from build123d import *

# Parameters (mm, degrees)
SKETCH_1_R      = 3
SKETCH_1_R_2    = 2
EXTRUDE_1_DEPTH = 3
FILLET_1_R      = 10
SKETCH_2_R      = 4
SKETCH_2_R_2    = 2
EXTRUDE_2_DEPTH = 10


with BuildPart() as part:
    # Эскиз1 → Бобышка-Вытянуть1 (new body)
    with BuildSketch(Plane.XY):
        with BuildLine():
            Line((-17.816178594, -6), (0, -6))
            ThreePointArc((0, -6), (6, 0), (0, 6))
            Line((0, 6), (-20, 6))
            ThreePointArc((-20, 6), (-22.05212086, 5.638155725), (-23.856725658, 4.596266659))
            Line((-23.856725658, 4.596266659), (-36.879481191, -6.331122706))
            ThreePointArc((-36.879481191, -6.331122706), (-37.619022192, -14.784115023), (-29.166029875, -15.523656023))
            Line((-29.166029875, -15.523656023), (-17.816178594, -6))
        make_face()
        with Locations((-20, 0)):
            Circle(SKETCH_1_R, mode=Mode.SUBTRACT)
        with BuildLine():
            Line((-6, 2), (0, 2))
            ThreePointArc((0, 2), (2, 0), (0, -2))
            Line((0, -2), (-6, -2))
            ThreePointArc((-6, -2), (-8, 0), (-6, 2))
        make_face(mode=Mode.SUBTRACT)
        with Locations((-33.022755533, -10.927389365)):
            Circle(SKETCH_1_R_2, mode=Mode.SUBTRACT)
    extrude(amount=EXTRUDE_1_DEPTH)

    # Скругление1
    fillet_1_edges = [part.edges().sort_by_distance(p)[0] for p in [
        (-17.816178594, -6, 1.5),
    ]]
    fillet(fillet_1_edges, radius=FILLET_1_R)

    # Эскиз2 → Бобышка-Вытянуть2 (add)
    with BuildSketch(Plane.XY.offset(3)):
        with Locations((-33.022755533, -10.927389365)):
            Circle(SKETCH_2_R)
        with Locations((-33.022755533, -10.927389365)):
            Circle(SKETCH_2_R_2, mode=Mode.SUBTRACT)
    extrude(amount=EXTRUDE_2_DEPTH)


solid = part.part
Geometry check sheet. Reference: the model listing, model coordinates, mm. A direction names the side the tool comes from. Round coordinates to 2 decimals unless told otherwise and drop trailing zeros. Loops run counter-clockwise (first coordinate to the right, second up) from the corner with the lowest first, then second, coordinate; pieces in that order, holes last. Notation, with made-up numbers: (14.25, 75.5) -> (24.25, 75.5) arc R8 ccw to (24.25, 90.5) -> close; hole circle Ø6 at (44.5, -8). An arc over 180 degrees is marked (long way). Answer as a JSON object with one key per item and string values. Group by question number.
Item 1: Cross-section at A-A, the plane x = -0.5. Record the cut outline in (y, z).
Item 2: Release check for a two-part mould opening along X. For faces 4 (the face through (-3, 2, 1)), 5 (the face through (2, 0, 1)), 6 (the face through (6, 0, 1)), 7 (the face through (-17, -3, 0)) record: pulls with the +X half, pulls with the -X half, needs draft (parallel to the pull), parting line crosses it, or undercut.
Item 3: Cross-section at B-B, the plane y = 0. Record the cut outline in (x, z), plus the area to 3 significant figures.
Item 4: Cross-section at C-C, the plane y = -10.25. Record the cut outline in (x, z).
Item 5: Thickness scan on line 1 along Y through (x, z) = (-6, 2); line 2 along X through (y, z) = (-0.5, 2.5); line 3 along Z through (x, y) = (-2.5, -2.5). Record the ranges inside material, lowest first.
Item 6: Cross-section at D-D, the plane z = 2.5. Record the cut outline in (x, y).
Item 7: Depth check by flat-ended pin: pin 1 Ø5 at (x, y) = (-16.5, -9) entering from +Z; pin 2 Ø6 at (x, y) = (-9.5, -1.5) entering from +Z; pin 3 Ø2.5 at (x, z) = (-4.5, 2) entering from -Y; pin 4 Ø4 at (y, z) = (-5.5, 8) entering from +X. Enter the tip coordinate at first touch or a pass-through.
Item 8: Set-up check for faces 1 (the face through (-8, 0, 1)), 2 (the face through (-29.33, -12.46, 7.93)), 3 (the face through (-7, -6, 1)): record each of +Z, -Z, +X, -X, +Y, -Y from which the full face is reachable in a straight line by a thin tool's end or side.
Determined:
{
 "1": {"outline": "(-6, 0) -> (-2, 0) -> (-2, 3) -> (-6, 3) -> close; (2, 0) -> (6, 0) -> (6, 3) -> (2, 3) -> close"},
 "2": {"face 4": "undercut", "face 5": "undercut", "face 6": "pulls with the +X half", "face 7": "needs draft"},
 "3": {"outline": "(-29.33, 0) -> (-23, 0) -> (-23, 3) -> (-29.33, 3) -> close; (-17, 0) -> (-8, 0) -> (-8, 3) -> (-17, 3) -> close; (2, 0) -> (6, 0) -> (6, 3) -> (2, 3) -> close", "area": "58.0 mm²"},
 "4": {"outline": "(-38.98, 0) -> (-34.9, 0) -> (-34.9, 13) -> (-36.96, 13) -> (-36.96, 3) -> (-38.98, 3) -> close; (-31.14, 0) -> (-22.88, 0) -> (-22.88, 3) -> (-29.08, 3) -> (-29.08, 13) -> (-31.14, 13) -> close"},
 "5": {"line 1": "y = -6 to -2, 2 to 6", "line 2": "x = -29.93 to -22.96, -17.04 to -7.94, 1.94 to 5.98", "line 3": "z = 0 to 3"},
 "6": {"outline": "(-36.88, -6.33) arc R6 ccw to (-29.17, -15.52) -> (-20.6, -8.34) arc R10 cw to (-14.18, -6) -> (0, -6) arc R6 ccw to (0, 6) -> (-20, 6) arc R6 ccw to (-23.86, 4.6) -> close; hole circle Ø4 at (-33.02, -10.93); hole circle Ø6 at (-20, 0); hole (-6, -2) -> (0, -2) arc R2 ccw to (0, 2) -> (-6, 2) arc R2 ccw to start"},
 "7": {"pin 1": "passes through", "pin 2": "stops at z = 3", "pin 3": "stops at y = -6", "pin 4": "stops at x = -30.96"},
 "8": {"face 1": "+Z, -Z", "face 2": "+Z", "face 3": "+Z, -Z, +X, -Y"}
}
